```python
from build123d import *

# Parameters (mm, degrees)
CORTE_EXTRUS_O1_DEPTH            = 20
FURO_DE_DI_METRO_27_0_27_1_D     = 27
FURO_DE_DI_METRO_27_0_27_1_DEPTH = 5
FURO_DE_DI_METRO_27_0_27_1_TIP   = 8.111618357
FILETE1_R                        = 4
CHANFRO1_SIZE                    = 3


with BuildPart() as part:
    # Esboço1 → Revolução1 (revolve)
    with BuildSketch(Plane.XY, mode=Mode.PRIVATE) as revolu_o1_sk:
        Polygon((0, 0), (0, 27), (36, 27), (36, 18), (156, 18), (156, 0), align=None)
    revolve(revolu_o1_sk.sketch.rotate(Axis((156, 0, 0), (-1, 0, 0)), 90), axis=Axis((156, 0, 0), (-1, 0, 0)))

    # Esboço2 → Corte-extrusão1 (cut)
    with BuildSketch(Plane.ZY):
        Polygon((0, 15.588457268), (-13.5, 7.794228634), (-13.5, -7.794228634), (0, -15.588457268), (13.5, -7.794228634), (13.5, 7.794228634), align=None)
    extrude(amount=-CORTE_EXTRUS_O1_DEPTH, mode=Mode.SUBTRACT)

    # Furo de diâmetro Ø27.0 (27)1
    with Locations(Plane.ZY.offset(-20)):
        with Locations((0, 0)):
            Hole(FURO_DE_DI_METRO_27_0_27_1_D / 2, depth=FURO_DE_DI_METRO_27_0_27_1_DEPTH)
            with Locations((0, 0, -(FURO_DE_DI_METRO_27_0_27_1_DEPTH + FURO_DE_DI_METRO_27_0_27_1_TIP / 2))):  # 118° drill point
                Cone(0, FURO_DE_DI_METRO_27_0_27_1_D / 2, FURO_DE_DI_METRO_27_0_27_1_TIP, mode=Mode.SUBTRACT)

    # Filete1
    filete1_edges = [part.edges().sort_by_distance(p)[0] for p in [
        (0, 0, 27),
    ]]
    fillet(filete1_edges, radius=FILETE1_R)

    # Chanfro1
    chanfro1_edges = [part.edges().sort_by_distance(p)[0] for p in [
        (156, 0, 18),
    ]]
    chamfer(chanfro1_edges, length=CHANFRO1_SIZE)


solid = part.part
```
Work out the finished part from the listing and answer in its coordinate system (mm). A direction names the side the tool comes from. Round coordinates to 2 decimals unless told otherwise and drop trailing zeros. Loops run counter-clockwise (first coordinate to the right, second up) from the corner with the lowest first, then second, coordinate; pieces in that order, holes last. Notation, with made-up numbers: M -21,79 L 15,79 A17 ccw 15,110 Z; hole C -38,-33.75 d2. An arc over 180 degrees is marked long. Use CSV: the item, a comma, the result in double quotes.
Q1. Each of these flat-tipped pins is pushed along its axis until it touches: pin 1 (2 mm diameter, centred on y = 21.5, z = 20, fed in from +X); pin 2 (1.2 mm diameter, centred on y = 13, z = 1.5, fed in from -X); pin 3 (3 mm diameter, centred on x = 107, z = -17.5, fed in from +Y); pin 4 (6 mm diameter, centred on x = 27.5, y = 7.5, fed in from +Z). Where does it stop, or does it pass through?
Determined:
pin 1,"through"
pin 2,"x = 20"
pin 3,"y = 8.25"
pin 4,"z = 26.62"
Q2. The mould has two halves that part along Y. Classify faces 1 (the flat face through (10, 0, -13.5)), 2 (the cylindrical face through (20.22, 26.36, 5.85)), 3 (the flat face through (156, 0, 0)): pulls with the +Y half, pulls with the -Y half, needs draft (parallel to the pull), parting line crosses it, or undercut.
Determined:
face 1,"undercut"
face 2,"parting line crosses it"
face 3,"needs draft"
Q3. Section A-A, the plane x = 86 is taken. Determine the outline of the cut face in (y, z), then the cut area to 3 significant figures.
Determined:
outline,"C 0,0 d36"
area,"1,020 mm2"
Q4. A tool of negligible diameter and unlimited length cuts with its end or side. For faces 4 (the flat face through (0, 10, 10)), 5 (the flat face through (20, 7, -12)), 6 (the flat face through (36, 18, -6)), from which of +Z, -Z, +X, -X, +Y, -Y can it reach the whole face along a straight path? Write none if from no direction.
Determined:
face 4,"+Z, -Z, -X, +Y, -Y"
face 5,"-X"
face 6,"+X"
Q5. Consider L1, parallel to Y at x = 22, z = 0; L2, parallel to X at y = -8, z = 22; L3, parallel to Y at x = 51, z = 1. Determine where each line is inside the solid, lowest interval first.
Determined:
L1,"-27 to -13.5, 13.5 to 27"
L2,"0.02 to 36"
L3,"-17.97 to 17.97"
